```python
from build123d import *

# Parameters (mm, degrees)
F0_W         = 40
F0_H         = 16
F1_DEPTH     = 4
F2_W         = 40
F2_H         = 4
F3_DEPTH     = 20
F4_D         = 6
F12_D        = 13
F6_SIZE      = 10
F8_DEPTH     = 2
F9_DEPTH     = 2
F10_T1_DEPTH = 29
F10_T3_DEPTH = 39
F11_R        = 10


# Not quite as in the source:
# - a fillet or chamfer that OpenCascade refuses, or shapes differently, is made with other operations: its cross-section is extruded or revolved along the edge and cut away or added


with BuildPart() as f1:
    # F0 (on Top) → F1 (new body)
    with BuildSketch(Plane.XY):
        Rectangle(F0_W, F0_H)
    extrude(amount=F1_DEPTH)

    # F2 (on face) → F3 (join)
    with BuildSketch(Plane.XY.offset(4)):
        with Locations((0, -6)):
            Rectangle(F2_W, F2_H)
    extrude(amount=F3_DEPTH)

    # F4 (through all)
    with Locations(Plane.XY.offset(4)):
        with Locations((-10, 0), (10, 0)):
            Hole(F4_D / 2)

    # F12 (through all)
    with Locations(Plane(origin=(0, -4, 0), x_dir=(-1, 0, 0), z_dir=(0, 1, 0))):
        with Locations((0, 14)):
            Hole(F12_D / 2)

    # F6
    f6_edges = [f1.edges().sort_by_distance(p)[0] for p in [
        (-20, -6, 24),
        (20, -6, 24),
    ]]
    chamfer(f6_edges, length=F6_SIZE)

    # F7 (on face) → F8 (join)
    with BuildSketch(Plane(origin=(-20, 0, 0), x_dir=(0, -1, 0), z_dir=(-1, 0, 0))):
        Polygon((4, 14), (-8, 4), (4, 4), align=None)
    extrude(amount=-F8_DEPTH)

    # F13 (on face) → F9 (join)
    with BuildSketch(Plane.YZ.offset(20)):
        Polygon((-4, 4), (8, 4), (-4, 14), align=None)
    extrude(amount=-F9_DEPTH)

    # F10: fillet of radius 5 on 4 edges, made by hand

    # F10_s2 → F10_t1 (cut)
    with BuildSketch(Plane.XY.offset(-12.5)):
        with BuildLine():
            ThreePointArc((20, 3), (18.5355339059, 6.5355339059), (15, 8))
            Line((15, 8), (20, 8))
            Line((20, 8), (20, 3))
        make_face()
        with BuildLine():
            ThreePointArc((-20, 3), (-18.5355339059, 6.5355339059), (-15, 8))
            Line((-15, 8), (-20, 8))
            Line((-20, 8), (-20, 3))
        make_face()
    extrude(amount=F10_T1_DEPTH, mode=Mode.SUBTRACT)

    # F10_s4 → F10_t3 (cut)
    with BuildSketch(Plane.XY.offset(-12.5)):
        with BuildLine():
            ThreePointArc((-15, -8), (-18.5355339059, -6.5355339059), (-20, -3))
            Line((-20, -3), (-20, -8))
            Line((-20, -8), (-15, -8))
        make_face()
        with BuildLine():
            ThreePointArc((15, -8), (18.5355339059, -6.5355339059), (20, -3))
            Line((20, -3), (20, -8))
            Line((20, -8), (15, -8))
        make_face()
    extrude(amount=F10_T3_DEPTH, mode=Mode.SUBTRACT)

    # F11
    f11_edges = [f1.edges().sort_by_distance(p)[0] for p in [
        (10, -6, 24),
        (-10, -6, 24),
    ]]
    fillet(f11_edges, radius=F11_R)


solid = f1.part
```
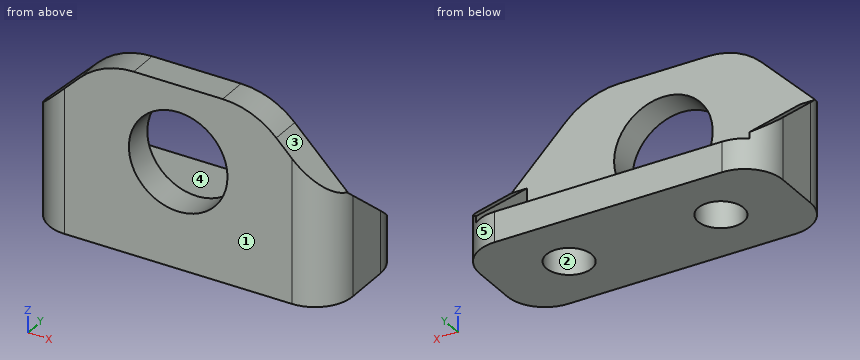
Design review of the part built by this model. Coordinates are the model's own, in mm. Face numbers are marked on the shaded views. A direction names the side the tool comes from. Coordinates: 2 decimals unless noted, no trailing zeros. Write each loop counter-clockwise with the first axis right and the second up, starting at its lowest first coordinate (ties: lowest second). Pieces come first, ordered by that corner, then holes. Notation, with made-up numbers: M 15.25,-31.75 L 55.25,-31.75 A14 ccw 55.25,-13.75 Z; hole C -22,72 d9. An arc over 180 degrees is marked long. Answer as a JSON object with one key per item and string values.
Item 1: Wall thickness on probe 1 along Z at (x, y) = (0, -5.2); probe 2 along X at (y, z) = (-0.75, 11); probe 3 along Z at (x, y) = (-17, -2): over which ranges is each line inside the solid? List them lowest first.
Outcome:
{"probe 1": "0 to 7.5, 20.5 to 24", "probe 2": "-20 to -18, 18 to 20", "probe 3": "0 to 4"}
Item 2: Insertion check: pin 1 Ø6 at (x, y) = (-5, 1.5) entering from +Z; pin 2 Ø6 at (x, z) = (2.5, 11) entering from +Y. Each pin has a flat end and moves straight along its axis. Give the tip position at first contact, or say it passes through.
Outcome:
{"pin 1": "z = 4", "pin 2": "y = -4"}
Item 3: Add section A-A, the plane x = 0. Give the boundary of the cut face in (y, z), and give its area (3 significant figures).
Outcome:
{"outline": "M -8,0 L 8,0 L 8,4 L -4,4 L -4,7.5 L -8,7.5 Z; M -8,20.5 L -4,20.5 L -4,24 L -8,24 Z", "area": "92.0 mm²"}
Item 4: Add section C-C, the plane z = 3.5. Give the boundary of the cut face in (x, y), and give its area (3 significant figures).
Outcome:
{"outline": "M -20,-3 A5 ccw -15,-8 L 15,-8 A5 ccw 20,-3 L 20,3 A5 ccw 15,8 L -15,8 A5 ccw -20,3 Z; hole C -10,0 d6; hole C 10,0 d6", "area": "562 mm²"}
Item 5: Add section B-B, the plane y = -7. Give the boundary of the cut face in (x, z), and give its area (3 significant figures).
Outcome:
{"outline": "M -18,0 L 18,0 L 18,16 L 12.93,21.07 A10 ccw 5.86,24 L -5.86,24 A10 ccw -12.93,21.07 L -18,16 Z; hole C 0,14 d13", "area": "663 mm²"}
Item 6: Machinability: for the marked faces 4 and 5, which of the approach directions +Z, -Z, +X, -X, +Y, -Y give a long, thin tool a straight path to every point of the face, cutting with its end or side? Answer none if there is none.
Outcome:
{"face 4": "+Z, +Y", "face 5": "+Z, -Z, +X, +Y"}
Item 7: Draft analysis for pull direction Y (two halves, no side actions). For the marked faces 1, 2 and 3, state which applies: pulls with the +Y half, pulls with the -Y half, needs draft (parallel to the pull), parting line crosses it, or undercut.
Outcome:
{"face 1": "pulls with the -Y half", "face 2": "undercut", "face 3": "needs draft"}
Item 8: Add section D-D, the plane z = 16.5. Give the boundary of the cut face in (x, y), and give its area (3 significant figures).
Outcome:
{"outline": "M -17.5,-7.33 A5 ccw -15,-8 L -6,-8 L -6,-4 L -17.5,-4 Z; M 6,-8 L 15,-8 A5 ccw 17.5,-7.33 L 17.5,-4 L 6,-4 Z", "area": "90.9 mm²"}
